```python
from build123d import *

# Parameters (mm, degrees)
SKETCH_1_W                       = 25
SKETCH_1_H                       = 66
SM_BASE_FLANGE_1_DEPTH           = 3
SM_EDGE_FLANGE_1_STRIP_W         = 13.4732
SM_EDGE_FLANGE_1_STRIP_H         = 3
SM_EDGE_FLANGE_1_STRIP_CUT_DEPTH = 66
SM_EDGE_FLANGE_1_DEPTH           = 66
HOLE_WIZARD_M8_1_D               = 6.8
HOLE_WIZARD_M6_2_D               = 5
OTHER_START                      = 9.5
OTHER_1_DEPTH                    = 3
OTHER_START_2                    = -3
OTHER_1_2_DEPTH                  = 3


# Read off the part's stored shape, not the designer's step: 断开-边角1
# Sheet-metal steps are written as plain solids
with BuildPart() as part:
    # Sketch 1 → 基体-法兰1 (new body)
    with BuildSketch(Plane.XY):
        Rectangle(SKETCH_1_W, SKETCH_1_H)
    extrude(amount=-SM_BASE_FLANGE_1_DEPTH)

    # 边线-法兰1 strip (across the edge) → 边线-法兰1 strip cut (cut)
    with BuildSketch(Plane(origin=(12.5, -33, 0), x_dir=(-1, 0, 0), z_dir=(0, 1, 0))):
        with Locations((-3, -1.5)):
            Rectangle(SM_EDGE_FLANGE_1_STRIP_W, SM_EDGE_FLANGE_1_STRIP_H)
    extrude(amount=SM_EDGE_FLANGE_1_STRIP_CUT_DEPTH, mode=Mode.SUBTRACT)

    # 边线-法兰1 section (across the edge) → 边线-法兰1 (add)
    with BuildSketch(Plane(origin=(12.5, -33, 0), x_dir=(-1, 0, 0), z_dir=(0, 1, 0))):
        with BuildLine():
            Line((0, 0.7366), (0, 15))
            Line((0, 15), (3, 15))
            Line((3, 15), (3, 0.7366))
            ThreePointArc((3, 0.7366), (3.215745145, 0.215745145), (3.7366, 0))
            Line((3.7366, 0), (3.7366, -3))
            ThreePointArc((3.7366, -3), (1.094424801, -1.905575199), (0, 0.7366))
        make_face()
    extrude(amount=SM_EDGE_FLANGE_1_DEPTH)

    # M8 螺纹孔1 (through all)
    with Locations(Plane.XY):
        with Locations((0, -20), (0, 20)):
            Hole(HOLE_WIZARD_M8_1_D / 2)

    # M6 螺纹孔2 (through all)
    with Locations(Plane.ZY.offset(-9.5)):
        with Locations((9, 0)):
            Hole(HOLE_WIZARD_M6_2_D / 2)

    # Other 1 outline → Other 1 (cut)
    with BuildSketch(Plane.YZ.offset(OTHER_START)):
        with BuildLine():
            Line((-33, 15), (-33, 12))
            ThreePointArc((-33, 12), (-32.121320344, 14.121320344), (-30, 15))
            Line((-30, 15), (-33, 15))
        make_face()
        with BuildLine():
            Line((33, 15), (30, 15))
            ThreePointArc((30, 15), (32.121320344, 14.121320344), (33, 12))
            Line((33, 12), (33, 15))
        make_face()
    extrude(amount=OTHER_1_DEPTH, mode=Mode.SUBTRACT)

    # Other 1 2 outline → Other 1 2 (cut)
    with BuildSketch(Plane.XY.offset(OTHER_START_2)):
        with BuildLine():
            Line((-12.5, 33), (-12.5, 30))
            ThreePointArc((-12.5, 30), (-11.621320344, 32.121320344), (-9.5, 33))
            Line((-9.5, 33), (-12.5, 33))
        make_face()
        with BuildLine():
            ThreePointArc((-9.5, -33), (-11.621320344, -32.121320344), (-12.5, -30))
            Line((-12.5, -30), (-12.5, -33))
            Line((-12.5, -33), (-9.5, -33))
        make_face()
    extrude(amount=OTHER_1_2_DEPTH, mode=Mode.SUBTRACT)


solid = part.part
```
For this review, take the finished solid that the model builds, in its own axes (mm). A direction names the side the tool comes from. Give positions to 0.01 mm unless a question says otherwise; leave off trailing zeros. Write each loop counter-clockwise with the first axis right and the second up, starting at its lowest first coordinate (ties: lowest second). Pieces come first, ordered by that corner, then holes.
Item 1: Machinability: for faces 1 (the face through (-2, 0, -3)), 2 (the face through (9.5, 0, 6)), which of the approach directions +Z, -Z, +X, -X, +Y, -Y give a long, thin tool a straight path to every point of the face, cutting with its end or side? Answer none if there is none.
Item 2: Wall thickness on probe 1 along Y at (x, z) = (0, -0.9); probe 2 along X at (y, z) = (13.5, 4.25); probe 3 along Y at (x, z) = (11.8, 9): over which ranges is each line inside the solid? List them lowest first.
Item 3: Insertion check: P1, Ø4, axis at x = -7.5, z = 3.5, coming from the -Y side; P2, Ø4, axis at y = 1.5, z = 10.5, coming from the -X side; P3, Ø11, axis at x = 0, y = 20, coming from the +Z side. Each pin has a flat end and moves straight along its axis. Give the tip position at first contact, or say it passes through.
Item 4: The part is to be moulded in two halves that separate along Y. For faces 3 (the face through (11, 0.1, 11.5)), 4 (the face through (12.5, 0, 6)), 5 (the face through (4.7, 33, -0.5)), say which applies: +Y half, -Y half, draft (parallel to the pull), parting line (faces both ways), or undercut.
Item 5: Take a section at C-C (z = 9). Give the boundary of the cut face in (x, y), and give its area (3 significant figures).
Item 6: Take a section at A-A (y = -20). Give the boundary of the cut face in (x, z).
Item 7: Take a section at D-D (y = 25). Give the boundary of the cut face in (x, z), and give its area (3 significant figures).
Item 8: Take a section at B-B (x = 0). Give the boundary of the cut face in (y, z), and give its area (3 significant figures).
Established:
1. face 1: -Z, +X, -X, +Y, -Y
1. face 2: +Z, -X, +Y, -Y
2. probe 1: y = -33 to -23.4, -16.6 to 16.6, 23.4 to 33
2. probe 2: x = 9.5 to 12.5
2. probe 3: y = -33 to -2.5, 2.5 to 33
3. P1: passes through
3. P2: stops at x = 9.5
3. P3: stops at z = 0
4. face 3: undercut
4. face 4: draft
4. face 5: +Y half
5. outline: (9.5, -33) - (12.5, -33) - (12.5, -2.5) - (9.5, -2.5) - close; (9.5, 2.5) - (12.5, 2.5) - (12.5, 33) - (9.5, 33) - close
5. area: 183 mm2
6. outline: (-12.5, -3) - (-3.4, -3) - (-3.4, 0) - (-12.5, 0) - close; (3.4, -3) - (8.76, -3) arc R3.74 ccw to (12.5, 0.74) - (12.5, 15) - (9.5, 15) - (9.5, 0.74) arc R0.74 cw to (8.76, 0) - (3.4, 0) - close
7. outline: (-12.5, -3) - (8.76, -3) arc R3.74 ccw to (12.5, 0.74) - (12.5, 15) - (9.5, 15) - (9.5, 0.74) arc R0.74 cw to (8.76, 0) - (-12.5, 0) - close
7. area: 117 mm2
8. outline: (-33, -3) - (-23.4, -3) - (-23.4, 0) - (-33, 0) - close; (-16.6, -3) - (16.6, -3) - (16.6, 0) - (-16.6, 0) - close; (23.4, -3) - (33, -3) - (33, 0) - (23.4, 0) - close
8. area: 157 mm2
